The figure shows three views and two pictorial views of one solid part (mm, origin at its lowest corner). Answer the questions. Give positions to 0.01 mm unless a question says otherwise; leave off trailing zeros. Loops run counter-clockwise (first coordinate to the right, second up) from the corner with the lowest first, then second, coordinate; pieces in that order, holes last.
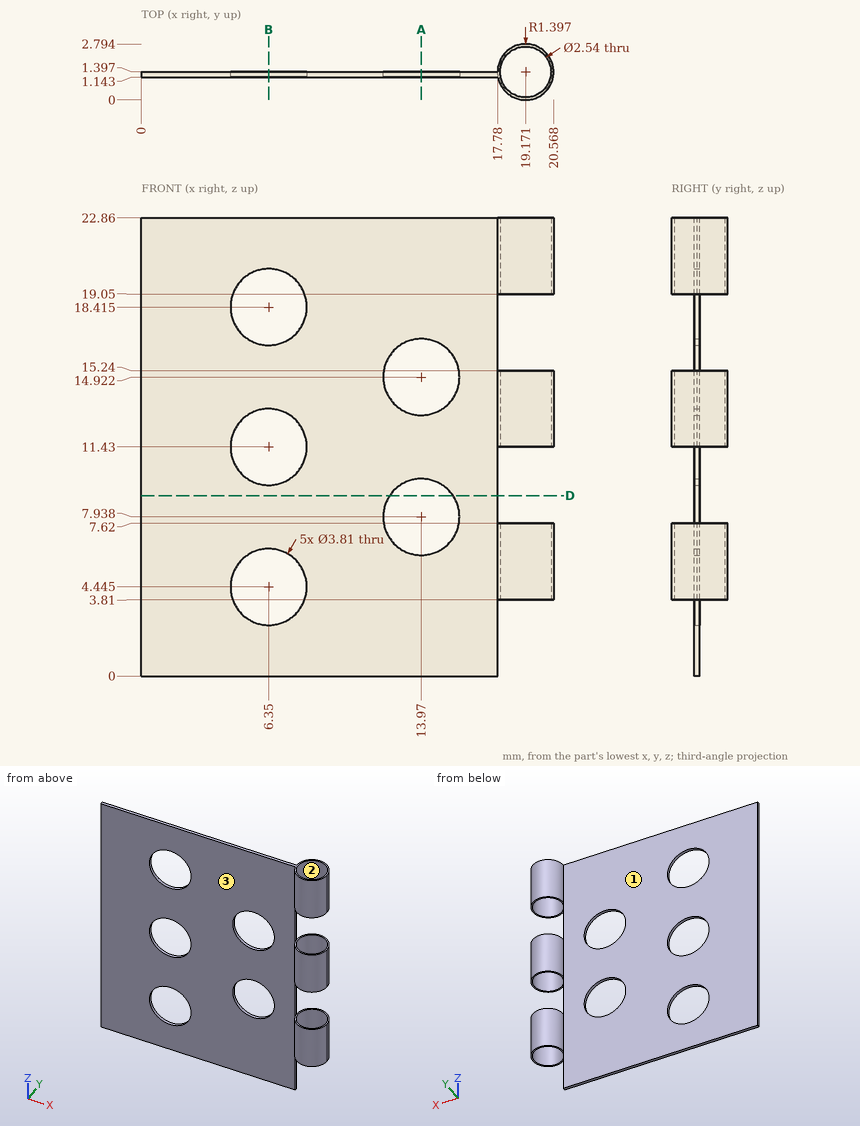
Q1. Given pin 1 (3 mm diameter, centred on x = 6.35, z = 11.43, fed in from -Y); pin 2 (6 mm diameter, centred on x = 2.5, z = 8.5, fed in from +Y); pin 3 (5.5 mm diameter, centred on x = 7.5, z = 8, fed in from -Y), each flat-ended and moving along its own axis, determine where each tip first touches the part or whether it passes through.
Q2. Determine the mould class of the marked faces 1, 2 and 3 for opening direction Y: +Y half, -Y half, draft (parallel to the pull), parting line (faces both ways), or undercut.
Q3. Section A-A on x = 13.97 is taken. Give the vertices of the cut face in (y, z).
Q4. Consider line 1 along Z through (x, y) = (13.97, 1.3); line 2 along Y through (x, z) = (5, 16); line 3 along X through (y, z) = (0.3, 4.25) (1 decimal). Determine where each line is inside the solid, lowest interval first.
Q5. Section D-D on z = 9 is taken. Give the vertices of the cut face in (x, y).
Q6. Section B-B on x = 6.35 is taken. State how many separate pieces and enclosed holes the cut face has.
Check result:
1. pin 1: passes through
1. pin 2: stops at y = 1.4
1. pin 3: stops at y = 1.14
2. face 1: +Y half
2. face 2: undercut
2. face 3: -Y half
3. outline: (1.14, 0) - (1.4, 0) - (1.4, 6.03) - (1.14, 6.03) - close; (1.14, 9.84) - (1.4, 9.84) - (1.4, 13.02) - (1.14, 13.02) - close; (1.14, 16.83) - (1.4, 16.83) - (1.4, 22.86) - (1.14, 22.86) - close
4. line 1: z = 0 to 6.03, 9.84 to 13.02, 16.83 to 22.86
4. line 2: y = 1.14 to 1.4
4. line 3: x = 18.3 to 18.5, 19.8 to 20
5. outline: (0, 1.14) - (12.39, 1.14) - (12.39, 1.4) - (0, 1.4) - close; (15.55, 1.14) - (17.78, 1.14) - (17.78, 1.4) - (15.55, 1.4) - close
6. separate pieces: 4
6. enclosed holes: 0
